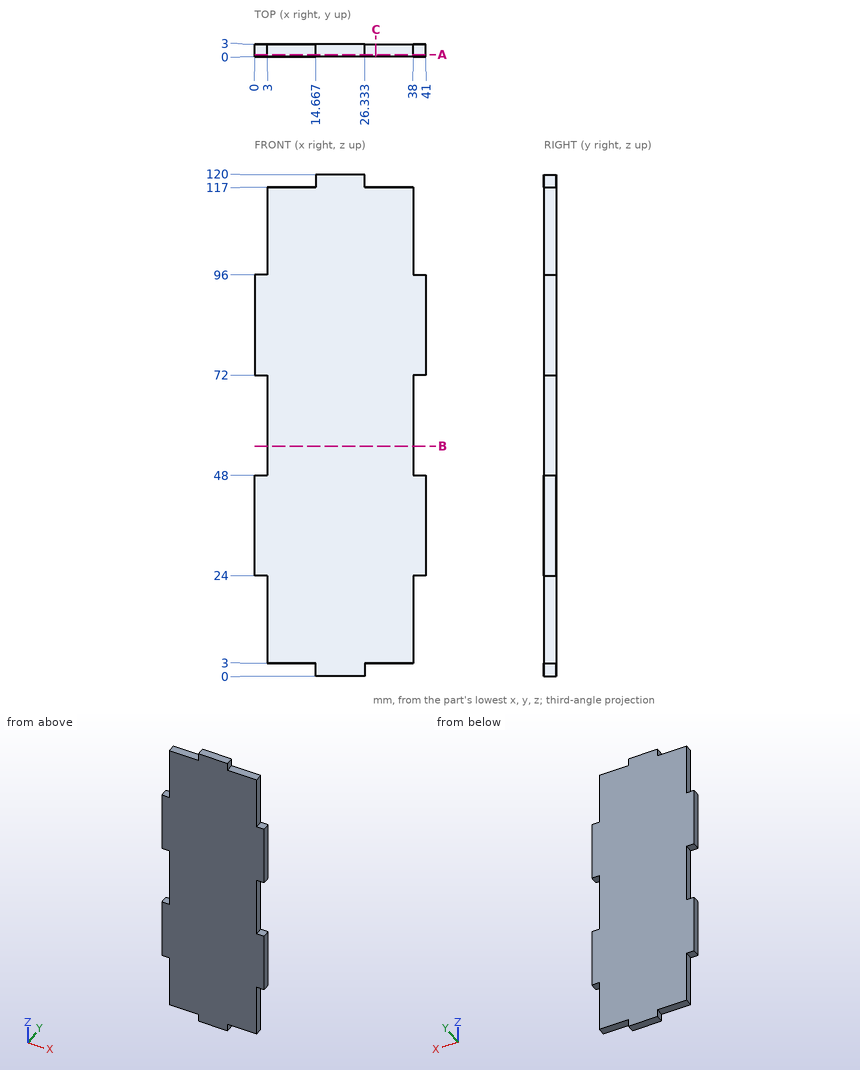
Answer from the drawing. Dimensions are ordinates in mm from the lowest x, y and z of the part. Round coordinates to 2 decimals unless told otherwise and drop trailing zeros. Loops run counter-clockwise (first coordinate to the right, second up) from the corner with the lowest first, then second, coordinate; pieces in that order, holes last. Notation, with made-up numbers: (-17.75, -30) - (25.25, -30) arc R21 cw to (25.25, -21) - close; hole circle Ø2 at (21, 2). An arc over 180 degrees is marked (long way). Return JSON: item names as keys, results as strings. Group by question number.
1. Each of these flat-tipped pins is pushed along its axis until it touches: P1, Ø1.5, axis at y = 2, z = 60, coming from the -X side; P2, Ø1.5, axis at x = 30, y = 1.5, coming from the -Z side; P3, Ø0.9, axis at x = 39, y = 2, coming from the +Z side. Where does it stop, or does it pass through?
2. The part is cut by section B-B on z = 55. Determine the outline of the cut face in (x, y), then the cut area to 3 significant figures.
3. The part is cut by section A-A on y = 0.45. Determine the outline of the cut face in (x, z).
4. Consider probe 1 along Z at (x, y) = (34, 2.35); probe 2 along Z at (x, y) = (39.5, 1.9); probe 3 along X at (y, z) = (0.5, 100). Determine where each line is inside the solid, lowest interval first.
5. The part is cut by section C-C on x = 29. Determine the outline of the cut face in (y, z).
Resolved:
{
 "1": {"P1": "stops at x = 3", "P2": "stops at z = 3", "P3": "stops at z = 96"},
 "2": {"outline": "(3, 0) - (38, 0) - (38, 3) - (3, 3) - close", "area": "105 mm²"},
 "3": {"outline": "(0, 24) - (3, 24) - (3, 3) - (14.67, 3) - (14.67, 0) - (26.33, 0) - (26.33, 3) - (38, 3) - (38, 24) - (41, 24) - (41, 48) - (38, 48) - (38, 72) - (41, 72) - (41, 96) - (38, 96) - (38, 117) - (26.33, 117) - (26.33, 120) - (14.67, 120) - (14.67, 117) - (3, 117) - (3, 96) - (0, 96) - (0, 72) - (3, 72) - (3, 48) - (0, 48) - close"},
 "4": {"probe 1": "z = 3 to 117", "probe 2": "z = 24 to 48, 72 to 96", "probe 3": "x = 3 to 38"},
 "5": {"outline": "(0, 3) - (3, 3) - (3, 117) - (0, 117) - close"}
}
